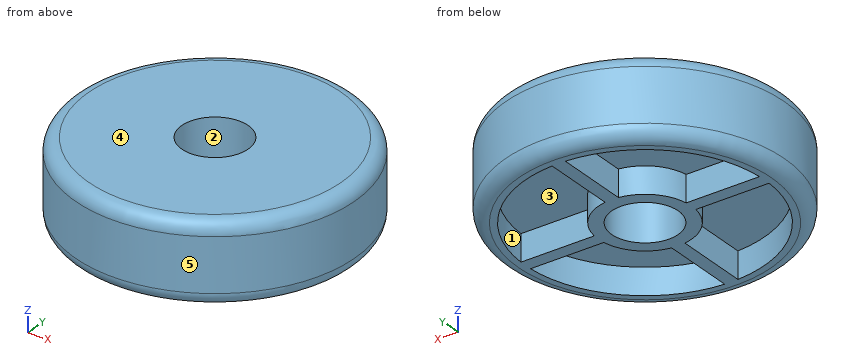
```python
from build123d import *

# Parameters (mm, degrees)
SKETCH1_R           = 10.5
BOSS_EXTRUDE1_DEPTH = 6
SKETCH2_R           = 2.5
CUT_EXTRUDE1_DEPTH  = 6
FILLET1_R           = 1
CUT_EXTRUDE2_DEPTH  = 2


with BuildPart() as part:
    # Sketch1 → Boss-Extrude1 (new body)
    with BuildSketch(Plane.XY):
        Circle(SKETCH1_R)
    extrude(amount=BOSS_EXTRUDE1_DEPTH)

    # Sketch2 → Cut-Extrude1 (cut)
    with BuildSketch(Plane(origin=(0, 0, 0), x_dir=(-1, 0, 0), z_dir=(0, 0, -1))):
        Circle(SKETCH2_R)
    extrude(amount=-CUT_EXTRUDE1_DEPTH, mode=Mode.SUBTRACT)

    # Fillet1
    fillet1_edges = [part.edges().sort_by_distance(p)[0] for p in [
        (-10.5, 0, 0),
        (-10.5, 0, 6),
    ]]
    fillet(fillet1_edges, radius=FILLET1_R)

    # Sketch3 → Cut-Extrude2 (cut)
    with BuildSketch(Plane(origin=(0, 0, 0), x_dir=(-1, 0, 0), z_dir=(0, 0, -1))):
        with BuildLine():
            Line((-0.5, 8.986100378), (-0.5, 3.464101615))
            ThreePointArc((-0.5, 3.464101615), (-2.474873734, 2.474873734), (-3.464101615, 0.5))
            Line((-3.464101615, 0.5), (-8.986100378, 0.5))
            ThreePointArc((-8.986100378, 0.5), (-6.363961031, 6.363961031), (-0.5, 8.986100378))
        make_face()
        with BuildLine():
            Line((0.5, 8.986100378), (0.5, 3.464101615))
            ThreePointArc((0.5, 3.464101615), (2.474873734, 2.474873734), (3.464101615, 0.5))
            Line((3.464101615, 0.5), (8.986100378, 0.5))
            ThreePointArc((8.986100378, 0.5), (6.363961031, 6.363961031), (0.5, 8.986100378))
        make_face()
        with BuildLine():
            Line((-8.986100378, -0.5), (-3.464101615, -0.5))
            ThreePointArc((-3.464101615, -0.5), (-2.474873734, -2.474873734), (-0.5, -3.464101615))
            Line((-0.5, -3.464101615), (-0.5, -8.986100378))
            ThreePointArc((-0.5, -8.986100378), (-6.363961031, -6.363961031), (-8.986100378, -0.5))
        make_face()
        with BuildLine():
            Line((0.5, -3.464101615), (0.5, -8.986100378))
            ThreePointArc((0.5, -8.986100378), (6.363961031, -6.363961031), (8.986100378, -0.5))
            Line((8.986100378, -0.5), (3.464101615, -0.5))
            ThreePointArc((3.464101615, -0.5), (2.474873734, -2.474873734), (0.5, -3.464101615))
        make_face()
    extrude(amount=-CUT_EXTRUDE2_DEPTH, mode=Mode.SUBTRACT)


solid = part.part
```
Design review of the part built by this model. Coordinates are the model's own, in mm. Face numbers are marked on the shaded views. A direction names the side the tool comes from. Coordinates: 2 decimals unless noted, no trailing zeros. Loops run counter-clockwise (first coordinate to the right, second up) from the corner with the lowest first, then second, coordinate; pieces in that order, holes last.
Q1. We need section C-C on z = 3.5. State the section outline as (x, y) points, and give its area (3 significant figures).
Reported:
outline: circle Ø21 at (0, 0); hole circle Ø5 at (0, 0)
area: 327 mm2
Q2. For pin 1 (1.6 mm diameter, centred on x = -7.5, z = 1, fed in from +Y); pin 2 (1.5 mm diameter, centred on x = 5.5, z = 5.5, fed in from +Y); pin 3 (1.5 mm diameter, centred on y = 3.5, z = 4.5, fed in from +X), all flat-tipped, find the tip position at first contact; note any pin that passes through.
Reported:
pin 1: stops at y = 8.08
pin 2: stops at y = 9.31
pin 3: stops at x = 10.13
Q3. We need section A-A on x = 0. State the section outline as (y, z) points, and give its area (3 significant figures).
Reported:
outline: (-10.5, 1) arc R1 ccw to (-9.5, 0) - (-2.5, 0) - (-2.5, 6) - (-9.5, 6) arc R1 ccw to (-10.5, 5) - close; (2.5, 0) - (9.5, 0) arc R1 ccw to (10.5, 1) - (10.5, 5) arc R1 ccw to (9.5, 6) - (2.5, 6) - close
area: 95.1 mm2
Q4. The part is to be moulded in two halves that separate along X. For the marked faces 3, 4 and 5, say which applies: +X half, -X half, draft (parallel to the pull), parting line (faces both ways), or undercut.
Reported:
face 3: undercut
face 4: draft
face 5: parting line
Q5. Tool access review of the marked faces 1 and 2: name each direction out of +Z, -Z, +X, -X, +Y, -Y from which nothing blocks a thin tool from reaching the whole face with its end or side.
Reported:
face 1: -Z
face 2: +Z, -Z
Q6. To check wall thickness, follow line 1 (Y direction, x = 0, z = 1.65); line 2 (X direction, y = 2, z = 0.5); line 3 (Y direction, x = -3.75, z = 0.9). State the ranges of each line that lie inside material, in increasing order.
Reported:
line 1: y = -10.5 to -2.5, 2.5 to 10.5
line 2: x = -10.17 to -8.77, -2.87 to -1.5, 1.5 to 2.87, 8.77 to 10.17
line 3: y = -9.8 to -8.18, -0.5 to 0.5, 8.18 to 9.8
